```python
from build123d import *

# Parameters (mm, degrees)
BOSS_EXTRUDE1_DEPTH = 5
FILLET1_R           = 3
FILLET2_R           = 6


with BuildPart() as part:
    # Sketch2 → Boss-Extrude1 (new body)
    with BuildSketch(Plane(origin=(0, 0, 0), x_dir=(1, 0, 0), z_dir=(0, 1, 0))):
        with BuildLine():
            ThreePointArc((-32.250789408, 12.414261501), (-27.5, 6.314261501), (-22.749210592, 12.414261501))
            Line((-22.749210592, 12.414261501), (-24.859924244, 12.414261501))
            ThreePointArc((-24.859924244, 12.414261501), (-27.5, 8.314261501), (-30.140075756, 12.414261501))
            Line((-30.140075756, 12.414261501), (-32.250789408, 12.414261501))
        make_face()
        with BuildLine():
            Line((25, 7), (25, 2.5))
            Line((25, 2.5), (-25, 2.5))
            Line((-25, 2.5), (-25, 7))
            ThreePointArc((-25, 7), (-27.5, 6.314261501), (-30, 7))
            Line((-30, 7), (-30, -2.5))
            Line((-30, -2.5), (30, -2.5))
            Line((30, -2.5), (30, 7))
            ThreePointArc((30, 7), (27.5, 6.314261501), (25, 7))
        make_face()
        with BuildLine():
            Line((30.140075756, 12.414261501), (32.250789408, 12.414261501))
            ThreePointArc((32.250789408, 12.414261501), (27.5, 6.314261501), (22.749210592, 12.414261501))
            Line((22.749210592, 12.414261501), (24.859924244, 12.414261501))
            ThreePointArc((24.859924244, 12.414261501), (27.5, 8.314261501), (30.140075756, 12.414261501))
        make_face()
    extrude(amount=BOSS_EXTRUDE1_DEPTH)

    # Fillet1
    fillet1_edges = [part.edges().sort_by_distance(p)[0] for p in [
        (-25, 2.5, -2.5),
        (25, 2.5, -2.5),
    ]]
    fillet(fillet1_edges, radius=FILLET1_R)

    # Fillet2
    fillet2_edges = [part.edges().sort_by_distance(p)[0] for p in [
        (30, 2.5, 2.5),
        (-30, 2.5, 2.5),
    ]]
    fillet(fillet2_edges, radius=FILLET2_R)


solid = part.part
```
For this review, take the finished solid that the model builds, in its own axes (mm). A direction names the side the tool comes from. Give positions to 0.01 mm unless a question says otherwise; leave off trailing zeros. Order: outer loops, then holes, each group sorted by start corner. A loop starts at its lowest first (then second) coordinate and runs counter-clockwise, first axis right, second up.
1) Insertion check: pin 1 (2.5 mm diameter, centred on x = -1, y = 2.5, fed in from -Z); pin 2 (1.8 mm diameter, centred on y = 3.5, z = -5.5, fed in from -X); pin 3 (3.5 mm diameter, centred on x = -27.5, z = -11.21, fed in from +Y); pin 4 (1.6 mm diameter, centred on y = 3.5, z = -6.5, fed in from +X). Each pin has a flat end and moves straight along its axis. Give the tip position at first contact, or say it passes through.
2) Take a section at A-A (z = -7.75). Give the boundary of the cut face in (x, y), then the cut area to 3 significant figures.
3) Take a section at C-C (x = 27.5). Give the boundary of the cut face in (y, z).
4) Wall thickness on line 1 (X direction, y = 3.4, z = -10); line 2 (X direction, y = 1.2, z = -10.75); line 3 (X direction, y = 4.35, z = -5.75): over which ranges is each line inside the solid? List them lowest first.
5) Take a section at B-B (y = 4.4). Give the boundary of the cut face in (x, z), then the cut area to 3 significant figures.
6) Take a section at D-D (z = 0). Give the boundary of the cut face in (x, y), then the cut area to 3 significant figures.
7) For faces 1 (the face through (0, 2, -2.5)), 2 (the face through (-30, 2, -5)), 3 (the face through (-25, 2, -6)), list the 3-axis set-ups (+Z, -Z, +X, -X, +Y, -Y) from which the entire face can be reached by the end or side of a thin tool; tool diameter is ignored.
8) The part is to be moulded in two halves that separate along X. For faces 4 (the face through (22.992, 2.465, -9.293)), 5 (the face through (30, 2, -5)), 6 (the face through (0, 2, 2.5)), say which applies: released by +X, released by -X, zero draft, split by the parting line, or undercut.
Derived:
1. pin 1: stops at z = -2.5
1. pin 2: stops at x = -30
1. pin 3: passes through
1. pin 4: stops at x = 30.45
2. outline: (-30.97, 0) - (-24.03, 0) - (-24.03, 5) - (-30.97, 5) - close; (24.03, 0) - (30.97, 0) - (30.97, 5) - (24.03, 5) - close
2. area: 69.3 mm2
3. outline: (0, -8.31) - (5, -8.31) - (5, 1.37) - (0, 1.37) - close
4. line 1: x = -32.25 to -30.13, -24.87 to -22.75, 22.75 to 24.87, 30.13 to 32.25
4. line 2: x = -32.38 to -30.36, -24.64 to -22.62, 22.62 to 24.64, 30.36 to 32.38
4. line 3: x = -30 to -25, 25 to 30
5. outline: (-32.25, -12.41) - (-30.14, -12.41) arc R2.9 cw (long way) to (-24.86, -12.41) - (-22.75, -12.41) arc R4.9 ccw to (-25, -7) - (-25, -5.5) arc R3 cw to (-22, -2.5) - (22, -2.5) arc R3 cw to (25, -5.5) - (25, -7) arc R4.9 ccw to (22.75, -12.41) - (24.86, -12.41) arc R2.9 cw (long way) to (30.14, -12.41) - (32.25, -12.41) arc R4.9 ccw to (30, -7) - (30, -3.5) arc R6 ccw to (24, 2.5) - (-24, 2.5) arc R6 ccw to (-30, -3.5) - (-30, -7) arc R4.9 ccw to start
5. area: 388 mm2
6. outline: (-28.87, 0) - (28.87, 0) - (28.87, 5) - (-28.87, 5) - close
6. area: 289 mm2
7. face 1: -Z, +Y, -Y
7. face 2: +Z, -X, +Y, -Y
7. face 3: +Y, -Y
8. face 4: undercut
8. face 5: released by +X
8. face 6: zero draft
